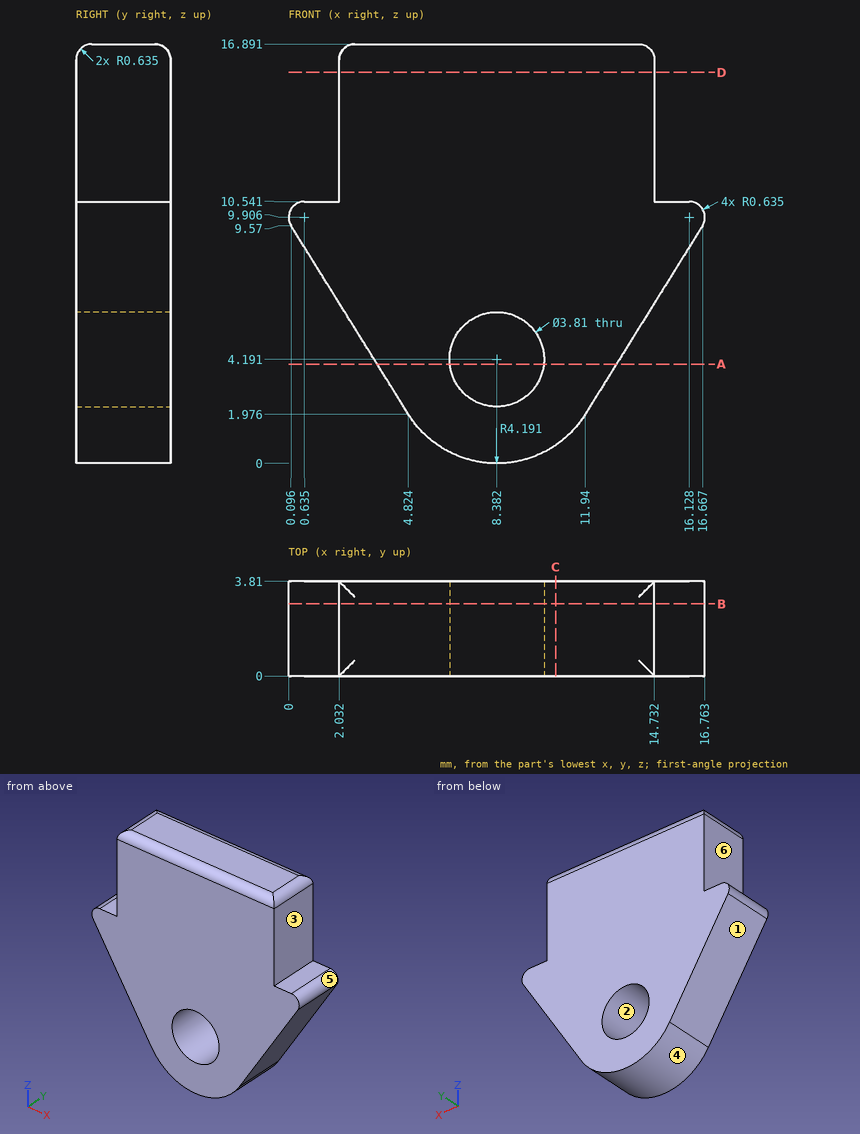
Geometry check sheet. Reference: drawing and pictorial views, mm from the part's lowest x, y, z. A direction names the side the tool comes from. Coordinates: 2 decimals unless noted, no trailing zeros. Write each loop counter-clockwise with the first axis right and the second up, starting at its lowest first coordinate (ties: lowest second). Pieces come first, ordered by that corner, then holes. Notation, with made-up numbers: (45.5, 33.25) -> (55.5, 33.25) arc R14 ccw to (55.5, 39.25) -> close; hole circle Ø4 at (-16.5, 38). An arc over 180 degrees is marked (long way). Use a Markdown table: item, result.
1. Tool access check on the marked faces 5 and 6. Record the directions out of +Z, -Z, +X, -X, +Y, -Y that give a thin tool (end or side, any length) a straight path to the whole face; none if there is none.
Reported:
| item | result |
|---|---|
| face 5 | +X, +Y, -Y |
| face 6 | +Z, -X, +Y, -Y |
2. Sectioned sample at C-C (x = 10.75). Enter the section's corners in (y, z) (1 decimal).
Reported:
| item | result |
|---|---|
| outline | (0, 0.7) -> (3.8, 0.7) -> (3.8, 16.3) arc R0.6 ccw to (3.2, 16.9) -> (0.6, 16.9) arc R0.6 ccw to (0, 16.3) -> close |
3. Sectioned sample at B-B (y = 2.9). Enter the section's corners in (x, z) (1 decimal), plus the area to 3 significant figures.
Reported:
| item | result |
|---|---|
| outline | (0.1, 9.6) -> (4.8, 2) arc R4.2 ccw to (11.9, 2) -> (16.7, 9.6) arc R0.6 ccw to (16.1, 10.5) -> (14.7, 10.5) -> (14.7, 16.3) arc R0.6 ccw to (14.1, 16.9) -> (2.7, 16.9) arc R0.6 ccw to (2, 16.3) -> (2, 10.5) -> (0.6, 10.5) arc R0.6 ccw to start; hole circle Ø3.8 at (8.4, 4.2) |
| area | 185 mm2 |
4. Scan lines: line 1 along X through (y, z) = (3.15, 15.75); line 2 along Z through (x, y) = (9, 1.3) (1 decimal); line 3 along Z through (x, y) = (10, 2.45) (1 decimal). Record each from-to range of solid material in increasing order.
Reported:
| item | result |
|---|---|
| line 1 | x = 2.03 to 14.73 |
| line 2 | z = 0 to 2.4, 6 to 16.9 |
| line 3 | z = 0.3 to 3.2, 5.2 to 16.9 |
5. Sectioned sample at D-D (z = 15.75). Enter the section's corners in (x, y).
Reported:
| item | result |
|---|---|
| outline | (2.03, 0) -> (14.73, 0) -> (14.73, 3.81) -> (2.03, 3.81) -> close |
6. Sectioned sample at A-A (z = 4). Enter the section's corners in (x, y).
Reported:
| item | result |
|---|---|
| outline | (3.56, 0) -> (6.49, 0) -> (6.49, 3.81) -> (3.56, 3.81) -> close; (10.28, 0) -> (13.2, 0) -> (13.2, 3.81) -> (10.28, 3.81) -> close |
7. Go/stop test with flat-tipped pins: pin 1 Ø1.5 at (x, y) = (1, 2) entering from +Z; pin 2 Ø1 at (x, y) = (6.5, 0.5) entering from -Z (1 decimal); pin 3 Ø1.9 at (y, z) = (3, 12) entering from -X. Record where each tip stops, or that it passes through.
Reported:
| item | result |
|---|---|
| pin 1 | stops at z = 10.54 |
| pin 2 | stops at z = 0.2 |
| pin 3 | stops at x = 2.03 |
8. Release check for a two-part mould opening along X. For the marked faces 1, 2, 3 and 4 record: pulls with the +X half, pulls with the -X half, needs draft (parallel to the pull), parting line crosses it, or undercut.
Reported:
| item | result |
|---|---|
| face 1 | pulls with the -X half |
| face 2 | undercut |
| face 3 | pulls with the +X half |
| face 4 | parting line crosses it |
